The figure shows three views and two pictorial views of one solid part (mm, origin at its lowest corner). Answer the questions. A direction names the side the tool comes from. Round coordinates to 2 decimals unless told otherwise and drop trailing zeros. Order: outer loops, then holes, each group sorted by start corner. A loop starts at its lowest first (then second) coordinate and runs counter-clockwise, first axis right, second up. Notation, with made-up numbers: M -35,20.25 L 14,20.25 A6 ccw 14,26.25 Z; hole C 56,1.25 d2. An arc over 180 degrees is marked long. Return JSON: item names as keys, results as strings.
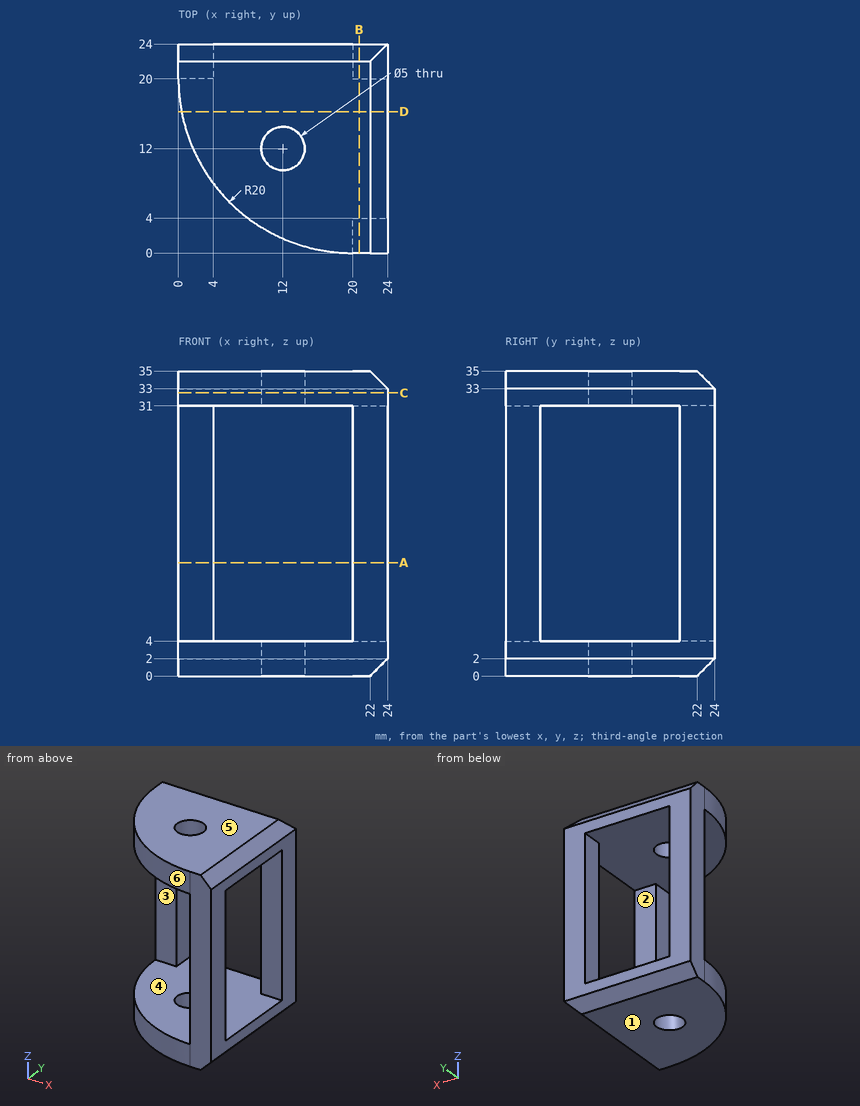
Item 1: The mould has two halves that part along X. Classify the marked faces 4, 5 and 6: pulls with the +X half, pulls with the -X half, needs draft (parallel to the pull), parting line crosses it, or undercut.
Output:
{"face 4": "undercut", "face 5": "needs draft", "face 6": "pulls with the -X half"}
Item 2: Find section B-B (x = 20.75). Determine the outline of the cut face in (y, z).
Output:
{"outline": "M 0,0 L 22,0 L 24,2 L 24,33 L 22,35 L 0,35 Z; hole M 4,4 L 20,4 L 20,31 L 4,31 Z"}
Item 3: Consider line 1 along Z through (x, y) = (20.25, 6); line 2 along X through (y, z) = (23.25, 10); line 3 along Z through (x, y) = (22.5, 14). Determine where each line is inside the solid, lowest interval first. Write a range as [from, to].
Output:
{"line 1": "z = [0, 4], [31, 35]", "line 2": "x = [0, 4], [20, 24]", "line 3": "z = [0.5, 4], [31, 34.5]"}
Item 4: Each of these flat-tipped pins is pushed along its axis until it touches: pin 1 (1.2 mm diameter, centred on x = 23, z = 21.5, fed in from -Y); pin 2 (1.2 mm diameter, centred on x = 1, z = 11.5, fed in from -Y); pin 3 (2 mm diameter, centred on y = 2.5, z = 17, fed in from -X). Where does it stop, or does it pass through?
Output:
{"pin 1": "stops at y = 0", "pin 2": "stops at y = 20", "pin 3": "stops at x = 20"}
Item 5: Find section D-D (y = 16.25). Determine the outline of the cut face in (x, z), plus the area to 3 significant figures.
Output:
{"outline": "M 0.35,0 L 22,0 L 24,2 L 24,4 L 0.35,4 Z; M 0.35,31 L 24,31 L 24,33 L 22,35 L 0.35,35 Z", "area": "185 mm^2"}
Item 6: Which of the six approach directions +Z, -Z, +X, -X, +Y, -Y give full straight-line access (tool end or side, diameter ignored) to the marked faces 1, 2 and 3?
Output:
{"face 1": "-Z, +X, -X, +Y, -Y", "face 2": "+X, -X", "face 3": "+X, -X, -Y"}
Item 7: Find section A-A (z = 13). Determine the outline of the cut face in (x, y), plus the area to 3 significant figures.
Output:
{"outline": "M 0,20 L 4,20 L 4,24 L 0,24 Z; M 20,0 L 24,0 L 24,4 L 20,4 Z; M 20,20 L 24,20 L 24,24 L 20,24 Z", "area": "48.0 mm^2"}
Item 8: Find section C-C (z = 32.5). Determine the outline of the cut face in (x, y), plus the area to 3 significant figures.
Output:
{"outline": "M 0,20 A20 ccw 20,0 L 24,0 L 24,24 L 0,24 Z; hole C 12,12 d5", "area": "471 mm^2"}
